For this review, take the finished solid that the model builds, in its own axes (mm). A direction names the side the tool comes from. Give positions to 0.01 mm unless a question says otherwise; leave off trailing zeros. Loops run counter-clockwise (first coordinate to the right, second up) from the corner with the lowest first, then second, coordinate; pieces in that order, holes last. Notation, with made-up numbers: (41.5, 88) -> (53.5, 88) arc R28 cw to (53.5, 126) -> close; hole circle Ø8 at (11.25, -18.75). An arc over 180 degrees is marked (long way). One line per question, with ' | ' between items. Start each with the question number.
(1) Tool access review of faces 4 (the flat face through (31, 140, -4)), 5 (the flat face through (25, 95, 14)), 6 (the flat face through (2, 24, 4)): name each direction out of +Z, -Z, +X, -X, +Y, -Y from which nothing blocks a thin tool from reaching the whole face with its end or side.
(2) Consider section A-A (y = 80). Write out the cut boundary in (x, z).
(3) Draft analysis for pull direction Z (two halves, no side actions). For faces 1 (the cylindrical face through (1.014, 42.727, 19.358)), 2 (the cylindrical face through (0.78, 49.177, 2.931)), 3 (the flat face through (26, 94, 16)), state which applies: +Z half, -Z half, draft (parallel to the pull), parting line (faces both ways), or undercut.
(4) Wall thickness on probe 1 along Z at (x, y) = (31.25, 80); probe 2 along Z at (x, y) = (28.5, 86); probe 3 along X at (y, z) = (72, -20): over which ranges is each line inside the solid? List them lowest first.
(5) Consider section C-C (z = 1). Write out the cut boundary in (x, y).
(6) Consider section D-D (z = 20.5). Write out the cut boundary in (x, y).
(7) Insertion check: P1, Ø1, axis at y = 77.5, z = -22.5, coming from the -X side; P2, Ø1.5, axis at x = 27.5, z = -15.5, coming from the -Y side; P3, Ø11, axis at y = 113.5, z = 2.5, coming from the -X side. Each pin has a flat end and moves straight along its axis. Give the tip position at first contact, or say it passes through.
(8) Consider section B-B (y = 40). Write out the cut boundary in (x, z), and give its area (3 significant figures).
from build123d import *

# Parameters (mm, degrees)
SM_BASE_FLANGE_1_DEPTH = 24
SKETCH_3_R             = 2.75
CUT_EXTRUDE_1_DEPTH    = 146.175755552
SKETCH_4_W             = 8
SKETCH_4_H             = 90
SKETCH_4_H_2           = 47.2634
CUT_EXTRUDE_2_DEPTH    = 146.602197786
CUT_EXTRUDE_3_DEPTH    = 99.488578018
SKETCH_9_W             = 2
SKETCH_9_H             = 89.2634
EXTRUDE_1_DEPTH        = 10
CHAMFER_1_SIZE         = 2
M4X0_7_1_D             = 3.3
M4X0_7_1_DEPTH         = 10.1
M4X0_7_1_TIP           = 0.991420021
SKETCH_12_R            = 8
CUT_EXTRUDE_4_DEPTH    = 99.488578018
SKETCH_13_R            = 2.75
CUT_EXTRUDE_5_DEPTH    = 146.175755552


# Sheet-metal steps are written as plain solids
with BuildPart() as part:
    # Sketch 1 → 基体-法兰1 (new, symmetric)
    with BuildSketch(Plane.XY):
        with BuildLine():
            Line((0, 0), (0, 47.2634))
            ThreePointArc((0, 47.2634), (0.801531583, 49.198468417), (2.7366, 50))
            Line((2.7366, 50), (29.2634, 50))
            ThreePointArc((29.2634, 50), (29.784254855, 50.215745145), (30, 50.7366))
            Line((30, 50.7366), (30, 140))
            Line((30, 140), (32, 140))
            Line((32, 140), (32, 50.7366))
            ThreePointArc((32, 50.7366), (31.198468417, 48.801531583), (29.2634, 48))
            Line((29.2634, 48), (2.7366, 48))
            ThreePointArc((2.7366, 48), (2.215745145, 47.784254855), (2, 47.2634))
            Line((2, 47.2634), (2, 0))
            Line((2, 0), (0, 0))
        make_face()
    extrude(amount=SM_BASE_FLANGE_1_DEPTH, both=True)

    # 草图3 → 切除-拉伸1 (cut, through all)
    with BuildSketch(Plane(origin=(2, 0, 0), x_dir=(0, 0, -1), z_dir=(1, 0, 0))):
        with Locations((-16, 6)):
            Circle(SKETCH_3_R)
        with Locations(Location((6, 6, 0), (0, 0, 180))):
            Circle(SKETCH_3_R)
    extrude(amount=-CUT_EXTRUDE_1_DEPTH, mode=Mode.SUBTRACT)

    # 草图4 → 切除-拉伸2 (cut, through all)
    with BuildSketch(Plane.ZY):
        with Locations((20, 95)):
            Rectangle(SKETCH_4_W, SKETCH_4_H)
        with Locations((-20, 23.6317)):
            Rectangle(SKETCH_4_W, SKETCH_4_H_2)
    extrude(amount=-CUT_EXTRUDE_2_DEPTH, mode=Mode.SUBTRACT)

    # 草图5 → 切除-拉伸3 (cut, through all)
    with BuildSketch(Plane(origin=(0, 50, 0), x_dir=(1, 0, 0), z_dir=(0, 1, 0))):
        Polygon((0, 24), (8, 24), (0, 16), align=None)
        Polygon((32, -16), (23.898364891, -24), (31.899002398, -24), align=None)
    extrude(amount=-CUT_EXTRUDE_3_DEPTH, mode=Mode.SUBTRACT)

    # 草图9 → 凸台-拉伸1 (add)
    with BuildSketch(Plane.ZY.offset(-30)):
        with Locations((-23, 95.3683)):
            Rectangle(SKETCH_9_W, SKETCH_9_H)
        with Locations((15, 95.3683)):
            Rectangle(SKETCH_9_W, SKETCH_9_H)
    extrude(amount=EXTRUDE_1_DEPTH)

    # 倒角1
    chamfer_1_edges = [part.edges().sort_by_distance(p)[0] for p in [
        (20, 140, -23),
        (20, 140, 15),
        (1, 0, 24),
        (1, 0, -16),
    ]]
    chamfer(chamfer_1_edges, length=CHAMFER_1_SIZE)

    # M4x0.7 螺纹孔1
    with Locations(Plane(origin=(32, 0, 0), x_dir=(0, 0, -1), z_dir=(1, 0, 0))):
        with Locations((-1, 80), (9, 80)):
            Hole(M4X0_7_1_D / 2, depth=M4X0_7_1_DEPTH)
            with Locations((0, 0, -(M4X0_7_1_DEPTH + M4X0_7_1_TIP / 2))):  # 118° drill point
                Cone(0, M4X0_7_1_D / 2, M4X0_7_1_TIP, mode=Mode.SUBTRACT)

    # 草图12 → 切除-拉伸4 (cut, through all)
    with BuildSketch(Plane(origin=(0, 50, 0), x_dir=(1, 0, 0), z_dir=(0, 1, 0))):
        with Locations(Location((16, 0, 0), (0, 0, 270))):
            Circle(SKETCH_12_R)
    extrude(amount=-CUT_EXTRUDE_4_DEPTH, mode=Mode.SUBTRACT)

    # 草图13 → 切除-拉伸5 (cut, through all)
    with BuildSketch(Plane(origin=(2, 0, 0), x_dir=(0, 0, -1), z_dir=(1, 0, 0))):
        with Locations((-19, 40)):
            Circle(SKETCH_13_R)
    extrude(amount=-CUT_EXTRUDE_5_DEPTH, mode=Mode.SUBTRACT)


solid = part.part
A:
1) face 4: +Z, -Z, +X, -X, +Y | face 5: -X, +Y | face 6: +Z, -Z, +X, -Y
2) outline: (20, -24) -> (32, -24) -> (32, -10.65) -> (30, -10.65) -> (30, -22) -> (20, -22) -> close; (20, 14) -> (30, 14) -> (30, 2.65) -> (32, 2.65) -> (32, 16) -> (20, 16) -> close; (30, -7.35) -> (32, -7.35) -> (32, -0.65) -> (30, -0.65) -> close
3) face 1: undercut | face 2: draft | face 3: +Z half
4) probe 1: z = -24 to -10.65, -7.35 to -0.65, 2.65 to 16 | probe 2: z = -24 to -22, 14 to 16 | probe 3: x = 30 to 32
5) outline: (0, 0) -> (2, 0) -> (2, 47.26) arc R0.74 cw to (2.74, 48) -> (8.06, 48) -> (8.06, 50) -> (2.74, 50) arc R2.74 ccw to (0, 47.26) -> close; (23.94, 48) -> (29.26, 48) arc R2.74 ccw to (32, 50.74) -> (32, 78.35) -> (30, 78.35) -> (30, 50.74) arc R0.74 cw to (29.26, 50) -> (23.94, 50) -> close; (30, 81.65) -> (32, 81.65) -> (32, 140) -> (30, 140) -> close
6) outline: (0, 0) -> (2, 0) -> (2, 37.7) -> (0, 37.7) -> close; (0, 42.3) -> (2, 42.3) -> (2, 47.26) arc R0.74 cw to (2.74, 48) -> (27.44, 48) -> (27.44, 50) -> (2.74, 50) arc R2.74 ccw to (0, 47.26) -> close
7) P1: stops at x = 20 | P2: stops at y = 48 | P3: stops at x = 30
8) outline: (0, -16) -> (2, -16) -> (2, 16.25) -> (0, 16.25) -> close; (0, 21.75) -> (2, 21.75) -> (2, 24) -> (0, 24) -> close | area: 69.0 mm^2
